The model under review builds one solid part; all positions refer to its coordinate system, in mm. A direction names the side the tool comes from. Coordinates: 2 decimals unless noted, no trailing zeros. Write each loop counter-clockwise with the first axis right and the second up, starting at its lowest first coordinate (ties: lowest second). Pieces come first, ordered by that corner, then holes.
```python
from build123d import *

# Parameters (mm, degrees)
SKETCH_W         = 35
SKETCH_H         = 25
PAD_DEPTH        = 20
POCKET_DEPTH     = 16
CHAMFER_SIZE2    = 14
CHAMFER_SIZE     = 4
CHAMFER001_SIZE2 = 14
CHAMFER001_SIZE  = 4
POCKET001_DEPTH  = 25.001


with BuildPart() as part:
    # Sketch → Pad (new body)
    with BuildSketch(Plane.XY):
        Rectangle(SKETCH_W, SKETCH_H)
    extrude(amount=PAD_DEPTH)

    # Sketch001 (on Face6 of Pad) → Pocket (cut)
    with BuildSketch(Plane.XY.offset(20)):
        Polygon((-12.25, -6.75), (12.25, -6.75), (12.25, 6.75), (-12.25, 6.75), (-12.25, 2.5), (-17.5, 2.5), (-17.5, -2.5), (-12.25, -2.5), align=None)
    extrude(amount=-POCKET_DEPTH, mode=Mode.SUBTRACT)

    # Chamfer
    chamfer_edges = [part.edges().sort_by_distance(p)[0] for p in [
        (0, -12.5, 20),
    ]]
    chamfer_side = part.faces().sort_by_distance((-17.069884, -7.5, 20))[0]
    chamfer(chamfer_edges, length=CHAMFER_SIZE, length2=CHAMFER_SIZE2, reference=chamfer_side)

    # Chamfer001
    chamfer001_edges = [part.edges().sort_by_distance(p)[0] for p in [
        (0, 12.5, 20),
    ]]
    chamfer001_side = part.faces().sort_by_distance((-17.091833, -5.5, 20))[0]
    chamfer(chamfer001_edges, length=CHAMFER001_SIZE, length2=CHAMFER001_SIZE2, reference=chamfer001_side)

    # Sketch002 (on Face6 of Chamfer001) → Pocket001 (cut, through all)
    with BuildSketch(Plane.XZ.offset(12.5)):
        Polygon((7.5, 20), (17.5, 20), (17.5, 6), align=None)
    extrude(amount=-POCKET001_DEPTH, mode=Mode.SUBTRACT)


solid = part.part
```
Item 1: For pin 1 (1.5 mm diameter, centred on x = -6.5, z = 10.5, fed in from -Y); pin 2 (2 mm diameter, centred on y = 3.5, z = 16, fed in from +X); pin 3 (3 mm diameter, centred on x = -13, z = 14.5, fed in from +Y), all flat-tipped, find the tip position at first contact; note any pin that passes through.
Solved:
pin 1: stops at y = -11.43
pin 2: stops at x = -12.25
pin 3: stops at y = 10.5
Item 2: Mouldability with a two-part tool opening along Y and no side actions: class faces 1 (the face through (0, 12.5, 3)), 2 (the face through (-12.25, -5, 12)), 3 (the face through (-8, 7, 20)) as pulls with the +Y half, pulls with the -Y half, needs draft (parallel to the pull), parting line crosses it, or undercut.
Solved:
face 1: pulls with the +Y half
face 2: undercut
face 3: needs draft
Item 3: Take a section at C-C, the plane z = 18.75. Write out the cut boundary in (x, y), plus the area to 3 significant figures.
Solved:
outline: (-17.5, -8.86) - (8.39, -8.86) - (8.39, -6.75) - (-12.25, -6.75) - (-12.25, -2.5) - (-17.5, -2.5) - close; (-17.5, 2.5) - (-12.25, 2.5) - (-12.25, 6.75) - (8.39, 6.75) - (8.39, 8.86) - (-17.5, 8.86) - close
area: 154 mm2
Item 4: To check wall thickness, follow line 1 along Y through (x, z) = (2.5, 4.75); line 2 along Z through (x, y) = (-9.5, 4); line 3 along Y through (x, z) = (6, 11). State the ranges of each line that lie inside material, in increasing order.
Solved:
line 1: y = -12.5 to -6.75, 6.75 to 12.5
line 2: z = 0 to 4
line 3: y = -11.07 to -6.75, 6.75 to 11.07
Item 5: Machinability: for faces 4 (the face through (12.25, 0, 9)), 5 (the face through (-15, -2.5, 12)), 6 (the face through (-4.13, -10.53, 12.9)), which of the approach directions +Z, -Z, +X, -X, +Y, -Y give a long, thin tool a straight path to every point of the face, cutting with its end or side? Answer none if there is none.
Solved:
face 4: +Z
face 5: +Z, -X
face 6: +Z, +X, -X, -Y
Item 6: Take a section at D-D, the plane y = -9. Write out the cut boundary in (x, z), plus the area to 3 significant figures.
Solved:
outline: (-17.5, 0) - (17.5, 0) - (17.5, 6) - (8.75, 18.25) - (-17.5, 18.25) - close
area: 585 mm2
Item 7: Take a section at A-A, the plane z = 4.75. Write out the cut boundary in (x, y).
Solved:
outline: (-17.5, -12.5) - (17.5, -12.5) - (17.5, 12.5) - (-17.5, 12.5) - (-17.5, 2.5) - (-12.25, 2.5) - (-12.25, 6.75) - (12.25, 6.75) - (12.25, -6.75) - (-12.25, -6.75) - (-12.25, -2.5) - (-17.5, -2.5) - close
Item 8: Take a section at B-B, the plane x = -14. Write out the cut boundary in (y, z).
Solved:
outline: (-12.5, 0) - (12.5, 0) - (12.5, 6) - (8.5, 20) - (2.5, 20) - (2.5, 4) - (-2.5, 4) - (-2.5, 20) - (-8.5, 20) - (-12.5, 6) - close
